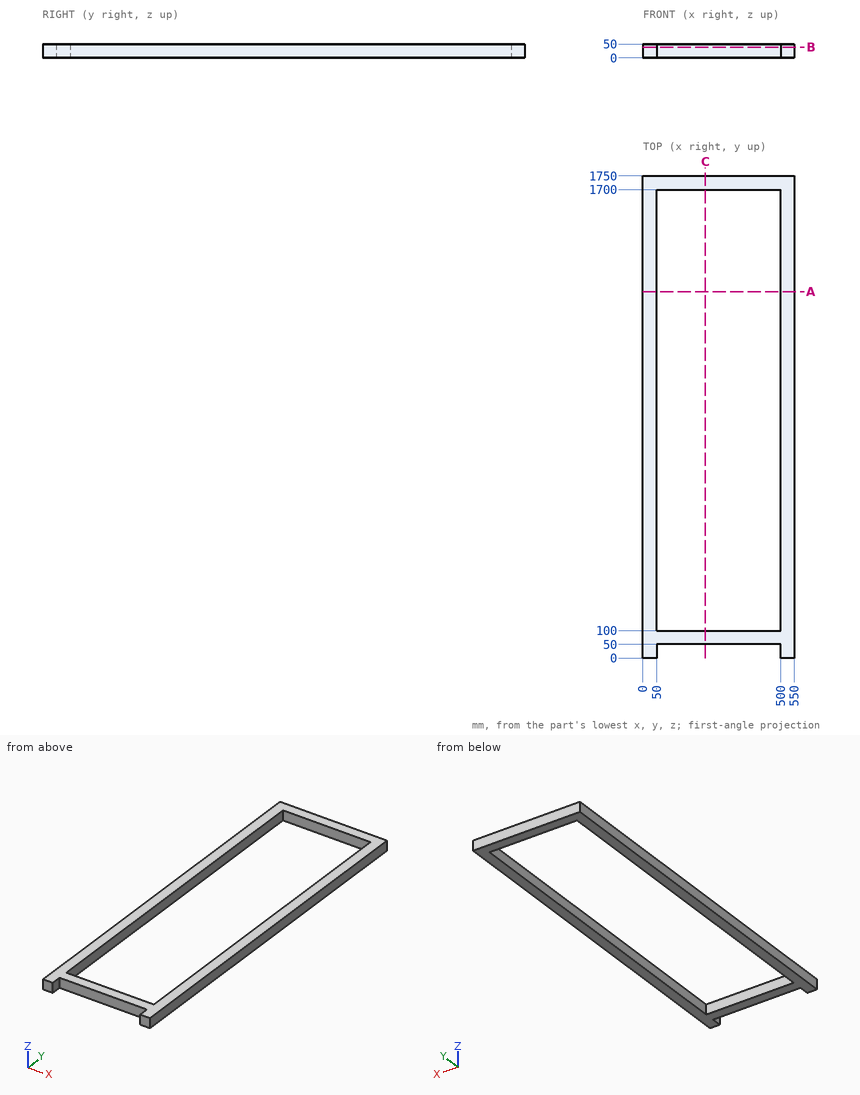
Geometry check sheet. Reference: drawing and pictorial views, mm from the part's lowest x, y, z. Give positions to 0.01 mm unless a question says otherwise; leave off trailing zeros. Order: outer loops, then holes, each group sorted by start corner. A loop starts at its lowest first (then second) coordinate and runs counter-clockwise, first axis right, second up. Notation, with made-up numbers: M 62.25,57.5 L 118.25,57.5 A23 cw 118.25,89.5 Z; hole C 5.25,62 d10. An arc over 180 degrees is marked long. Answer as a JSON object with one key per item and string values. Group by question number.
1) Cross-section at C-C (x = 226.5). Enter the section's corners in (y, z), then the cut area to 3 significant figures.
2) Cross-section at B-B (z = 38.5). Enter the section's corners in (x, y), then the cut area to 3 significant figures.
3) Depth check by flat-ended pin: pin 1 Ø6 at (x, z) = (195.5, 14) entering from -Y. Enter the tip coordinate at first touch or a pass-through.
4) Scan lines: line 1 along Y through (x, z) = (292.5, 18.5); line 2 along X through (y, z) = (1560, 22). Record each from-to range of solid material in increasing order. Write a range as [from, to].
5) Cross-section at A-A (y = 1330). Enter the section's corners in (x, z).
Result sheet:
{
 "1": {"outline": "M 50,0 L 100,0 L 100,50 L 50,50 Z; M 1700,0 L 1750,0 L 1750,50 L 1700,50 Z", "area": "5,000 mm2"},
 "2": {"outline": "M 0,0 L 50,0 L 50,50 L 500,50 L 500,0 L 550,0 L 550,1750 L 0,1750 Z; hole M 50,100 L 500,100 L 500,1700 L 50,1700 Z", "area": "220,000 mm2"},
 "3": {"pin 1": "stops at y = 50"},
 "4": {"line 1": "y = [50, 100], [1700, 1750]", "line 2": "x = [0, 50], [500, 550]"},
 "5": {"outline": "M 0,0 L 50,0 L 50,50 L 0,50 Z; M 500,0 L 550,0 L 550,50 L 500,50 Z"}
}
